Build history of the part. All positions in model axes, mm. A direction names the side the tool comes from. Round coordinates to 2 decimals unless told otherwise and drop trailing zeros. Loops run counter-clockwise (first coordinate to the right, second up) from the corner with the lowest first, then second, coordinate; pieces in that order, holes last. Notation, with made-up numbers: (25.25, 41.5) - (53.25, 41.5) arc R7 ccw to (53.25, 46.5) - close; hole circle Ø6 at (80.5, 37.5). An arc over 180 degrees is marked (long way). Use a Markdown table: item, result.
from build123d import *

# Parameters (mm, degrees)
CROQUIS1_W              = 70.8
CROQUIS1_H              = 48
CROQUIS1_W_2            = 60.4
CROQUIS1_H_2            = 44
CROQUIS1_W_3            = 59.6
CROQUIS1_H_3            = 43.2
CROQUIS1_W_4            = 43.2
CROQUIS1_H_4            = 27
SALIENTE_EXTRUIR1_DEPTH = 1.6
SALIENTE_EXTRUIR2_DEPTH = 10.8
CROQUIS1_5_W            = 70.8
CROQUIS1_5_H            = 48
CROQUIS1_5_W_2          = 60.4
CROQUIS1_5_H_2          = 44
CROQUIS1_5_W_3          = 59.6
CROQUIS1_5_H_3          = 43.2
SALIENTE_EXTRUIR3_DEPTH = 2.6
CORTAR_EXTRUIR1_REACH   = 77.533


with BuildPart() as part:
    # Croquis1 → Saliente-Extruir1 (new body)
    # profile 1 of 7: a face of its own
    with BuildSketch(Plane(origin=(0, 0, 0), x_dir=(1, 0, 0), z_dir=(0, 1, 0))):
        Rectangle(CROQUIS1_W, CROQUIS1_H)
        Rectangle(CROQUIS1_W_2, CROQUIS1_H_2, mode=Mode.SUBTRACT)
    # profile 2 of 7: a face of its own
    with BuildSketch(Plane(origin=(0, 0, 0), x_dir=(1, 0, 0), z_dir=(0, 1, 0))):
        Rectangle(CROQUIS1_W_2, CROQUIS1_H_2)
        Rectangle(CROQUIS1_W_3, CROQUIS1_H_3, mode=Mode.SUBTRACT)
    # profile 3 of 7: a face of its own
    with BuildSketch(Plane(origin=(0, 0, 0), x_dir=(1, 0, 0), z_dir=(0, 1, 0))):
        with BuildLine():
            ThreePointArc((-29.8, -16.4), (-26.123044738, -17.923044738), (-24.6, -21.6))
            Line((-24.6, -21.6), (24.6, -21.6))
            ThreePointArc((24.6, -21.6), (26.123044738, -17.923044738), (29.8, -16.4))
            Line((29.8, -16.4), (29.8, 16.4))
            ThreePointArc((29.8, 16.4), (26.123044738, 17.923044738), (24.6, 21.6))
            Line((24.6, 21.6), (-24.6, 21.6))
            ThreePointArc((-24.6, 21.6), (-26.123044738, 17.923044738), (-29.8, 16.4))
            Line((-29.8, 16.4), (-29.8, -16.4))
        make_face()
        with Locations((0, -2)):
            Rectangle(CROQUIS1_W_4, CROQUIS1_H_4, mode=Mode.SUBTRACT)
    # profile 4 of 7: a face of its own
    with BuildSketch(Plane(origin=(0, 0, 0), x_dir=(1, 0, 0), z_dir=(0, 1, 0))):
        with BuildLine():
            ThreePointArc((29.8, -16.4), (26.123044738, -17.923044738), (24.6, -21.6))
            Line((24.6, -21.6), (29.8, -21.6))
            Line((29.8, -21.6), (29.8, -16.4))
        make_face()
    # profile 5 of 7: a face of its own
    with BuildSketch(Plane(origin=(0, 0, 0), x_dir=(1, 0, 0), z_dir=(0, 1, 0))):
        with BuildLine():
            ThreePointArc((24.6, 21.6), (26.123044738, 17.923044738), (29.8, 16.4))
            Line((29.8, 16.4), (29.8, 21.6))
            Line((29.8, 21.6), (24.6, 21.6))
        make_face()
    # profile 6 of 7: a face of its own
    with BuildSketch(Plane(origin=(0, 0, 0), x_dir=(1, 0, 0), z_dir=(0, 1, 0))):
        with BuildLine():
            Line((-29.8, 21.6), (-29.8, 16.4))
            ThreePointArc((-29.8, 16.4), (-26.123044738, 17.923044738), (-24.6, 21.6))
            Line((-24.6, 21.6), (-29.8, 21.6))
        make_face()
    # profile 7 of 7: a face of its own
    with BuildSketch(Plane(origin=(0, 0, 0), x_dir=(1, 0, 0), z_dir=(0, 1, 0))):
        with BuildLine():
            Line((-29.8, -16.4), (-29.8, -21.6))
            Line((-29.8, -21.6), (-24.6, -21.6))
            ThreePointArc((-24.6, -21.6), (-26.123044738, -17.923044738), (-29.8, -16.4))
        make_face()
    extrude(amount=SALIENTE_EXTRUIR1_DEPTH)

    # Croquis1<4> → Saliente-Extruir2 (add)
    with BuildSketch(Plane(origin=(0, 0, 0), x_dir=(1, 0, 0), z_dir=(0, 1, 0))):
        with BuildLine():
            Line((-29.8, -16.4), (-29.8, -21.6))
            Line((-29.8, -21.6), (-24.6, -21.6))
            ThreePointArc((-24.6, -21.6), (-26.123044738, -17.923044738), (-29.8, -16.4))
        make_face()
        with BuildLine():
            Line((-29.8, 21.6), (-29.8, 16.4))
            ThreePointArc((-29.8, 16.4), (-26.123044738, 17.923044738), (-24.6, 21.6))
            Line((-24.6, 21.6), (-29.8, 21.6))
        make_face()
        with BuildLine():
            ThreePointArc((24.6, 21.6), (26.123044738, 17.923044738), (29.8, 16.4))
            Line((29.8, 16.4), (29.8, 21.6))
            Line((29.8, 21.6), (24.6, 21.6))
        make_face()
        with BuildLine():
            ThreePointArc((29.8, -16.4), (26.123044738, -17.923044738), (24.6, -21.6))
            Line((24.6, -21.6), (29.8, -21.6))
            Line((29.8, -21.6), (29.8, -16.4))
        make_face()
    extrude(amount=-SALIENTE_EXTRUIR2_DEPTH)

    # Croquis1<5> → Saliente-Extruir3 (add)
    # profile 1 of 2: a face of its own
    with BuildSketch(Plane(origin=(0, 0, 0), x_dir=(1, 0, 0), z_dir=(0, 1, 0))):
        Rectangle(CROQUIS1_5_W, CROQUIS1_5_H)
        Rectangle(CROQUIS1_5_W_2, CROQUIS1_5_H_2, mode=Mode.SUBTRACT)
    # profile 2 of 2: a face of its own
    with BuildSketch(Plane(origin=(0, 0, 0), x_dir=(1, 0, 0), z_dir=(0, 1, 0))):
        Rectangle(CROQUIS1_5_W_2, CROQUIS1_5_H_2)
        Rectangle(CROQUIS1_5_W_3, CROQUIS1_5_H_3, mode=Mode.SUBTRACT)
    extrude(amount=-SALIENTE_EXTRUIR3_DEPTH)

    # Cortar-Extruir1: up to this face of the body (flat: up to its plane)
    cortar_extruir1_end = Plane(part.part.faces().sort_by_distance((-35.4, -0.5, 0))[0])
    # Croquis2 → Cortar-Extruir1 (cut, up to the picked face)
    with BuildSketch(Plane(origin=(35.4, 0, 0), x_dir=(0, 0, -1), z_dir=(1, 0, 0)), mode=Mode.PRIVATE) as cortar_extruir1_sk1:
        with BuildLine():
            Line((-2.6, -2.6), (2.6, -2.6))
            ThreePointArc((2.6, -2.6), (0, 0), (-2.6, -2.6))
        make_face()
    cortar_extruir1_tool1 = split(extrude(cortar_extruir1_sk1.sketch, amount=-CORTAR_EXTRUIR1_REACH, mode=Mode.PRIVATE), bisect_by=cortar_extruir1_end, keep=Keep.BOTH, mode=Mode.PRIVATE)
    add(cortar_extruir1_tool1.solids().sort_by(Axis((35.4, -1.496526, 0), (-1, 0, 0)))[0], mode=Mode.SUBTRACT)


solid = part.part
Q1. Cut at C-C, the plane x = 13.5. List the corners of the cut face in (y, z).
Results found:
| item | result |
|---|---|
| outline | (-2.6, -24) - (1.6, -24) - (1.6, -11.5) - (0, -11.5) - (0, -21.6) - (-2.6, -21.6) - close; (-2.6, 21.6) - (0, 21.6) - (0, 15.5) - (1.6, 15.5) - (1.6, 24) - (-2.6, 24) - close |
Q2. Cut at B-B, the plane y = -9. List the corners of the cut face in (x, z), plus the area to 3 significant figures.
Results found:
| item | result |
|---|---|
| outline | (-29.8, -21.6) - (-24.6, -21.6) arc R5.2 ccw to (-29.8, -16.4) - close; (-29.8, 16.4) arc R5.2 ccw to (-24.6, 21.6) - (-29.8, 21.6) - close; (24.6, -21.6) - (29.8, -21.6) - (29.8, -16.4) arc R5.2 ccw to start; (24.6, 21.6) arc R5.2 ccw to (29.8, 16.4) - (29.8, 21.6) - close |
| area | 84.9 mm2 |
Q3. Probe line 1 (Z direction, x = 7.5, y = -1.75); line 2 (X direction, y = -2, z = -7.5); line 3 (Z direction, x = 1, y = 0.5). List the from-to ranges inside material, lowest first.
Results found:
| item | result |
|---|---|
| line 1 | z = -24 to -21.6, 21.6 to 24 |
| line 2 | x = -35.4 to -29.8, 29.8 to 35.4 |
| line 3 | z = -24 to -11.5, 15.5 to 24 |
Q4. Cut at D-D, the plane z = -20. List the corners of the cut face in (x, y), plus the area to 3 significant figures.
Results found:
| item | result |
|---|---|
| outline | (-35.4, -2.6) - (-29.8, -2.6) - (-29.8, -10.8) - (-24.85, -10.8) - (-24.85, 0) - (24.85, 0) - (24.85, -10.8) - (29.8, -10.8) - (29.8, -2.6) - (35.4, -2.6) - (35.4, 1.6) - (-35.4, 1.6) - close |
| area | 249 mm2 |
Q5. Pull direction Z, two halves, no side cores. Call faces 5 (the face through (29.8, -7, -19)), 6 (the face through (0, 1, 15.5)), 7 (the face through (27, -7, 21.6)): pulls with the +Z half, pulls with the -Z half, needs draft (parallel to the pull), parting line crosses it, or undercut.
Results found:
| item | result |
|---|---|
| face 5 | needs draft |
| face 6 | undercut |
| face 7 | pulls with the +Z half |
Q6. Which spindle directions (+Z, -Z, +X, -X, +Y, -Y) get a long thin tool onto all of the face, cutting with end or side? Do faces 1 (the face through (-29.8, -7, -19)), 2 (the face through (35.4, 0.5, 0.3)), 3 (the face through (0, 1, -11.5)), 4 (the face through (29.8, -1, 8)). Say none if no direction does.
Results found:
| item | result |
|---|---|
| face 1 | +Z, -Z, -X, -Y |
| face 2 | +Z, -Z, +X, +Y, -Y |
| face 3 | +Y, -Y |
| face 4 | -Y |
Q7. Cut at A-A, the plane z = 11. List the corners of the cut face in (x, y), plus the area to 3 significant figures.
Results found:
| item | result |
|---|---|
| outline | (-35.4, -2.6) - (-29.8, -2.6) - (-29.8, 0) - (-21.6, 0) - (-21.6, 1.6) - (-35.4, 1.6) - close; (21.6, 0) - (29.8, 0) - (29.8, -2.6) - (35.4, -2.6) - (35.4, 1.6) - (21.6, 1.6) - close |
| area | 73.3 mm2 |
Q8. Drop flat-ended pins along their axis: pin 1 (17 mm diameter, centred on x = 10.5, z = 14.5, fed in from -Y); pin 2 (21.5 mm diameter, centred on x = -14.5, z = 0, fed in from -Y); pin 3 (2.5 mm diameter, centred on x = 28, y = -7, fed in from +Z). Give the stop position or say it passes through.
Results found:
| item | result |
|---|---|
| pin 1 | stops at y = -2.6 |
| pin 2 | stops at y = 0 |
| pin 3 | stops at z = 21.6 |
